Here's how the part is built. I have some questions about the finished solid (model axes, mm). Face numbers are marked on the shaded views. A direction names the side the tool comes from. Coordinates: 2 decimals unless noted, no trailing zeros.
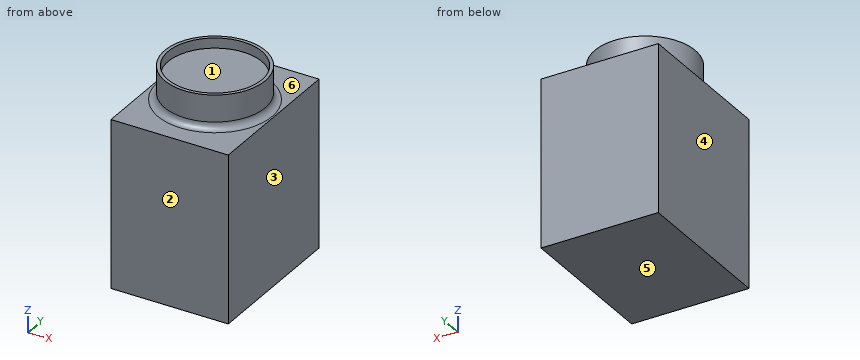
from build123d import *

# Parameters (mm, degrees)
SKETCH_W     = 35
SKETCH_H     = 45
PAD_DEPTH    = 50
SKETCH001_R  = 15
PAD001_DEPTH = 10
SKETCH002_R  = 14
POCKET_DEPTH = 3
FILLET_R     = 2


with BuildPart() as part:
    # Sketch → Pad (new body)
    with BuildSketch(Plane.XY):
        with Locations((2.787933, 6.169585)):
            Rectangle(SKETCH_W, SKETCH_H)
    extrude(amount=PAD_DEPTH)

    # Sketch001 (on Face6 of Pad) → Pad001 (join)
    with BuildSketch(Plane.XY.offset(50)):
        with Locations((2.787933, 6.169585)):
            Circle(SKETCH001_R)
    extrude(amount=PAD001_DEPTH)

    # Sketch002 (on Face8 of Pad001) → Pocket (cut)
    with BuildSketch(Plane.XY.offset(60)):
        with Locations((2.787933, 6.169585)):
            Circle(SKETCH002_R)
    extrude(amount=-POCKET_DEPTH, mode=Mode.SUBTRACT)

    # Fillet
    fillet_edges = [part.edges().sort_by_distance(p)[0] for p in [
        (-12.212067, 6.169585, 50),
    ]]
    fillet(fillet_edges, radius=FILLET_R)


solid = part.part
1. If I drill on line 1 (Z direction, x = 9, y = 1); line 2 (Z direction, x = 8, y = 26); line 3 (X direction, y = 5.5, z = 53.5), over which ranges is the centre line in solid material (lowest first)?
2. On a 3-axis mill with a long thin cutter (end or side, diameter ignored), from which of +Z, -Z, +X, -X, +Y, -Y can I reach the whole of each face in a straight line? I mean the marked faces 5 and 6. Say none if no direction works.
3. Thinking about a two-plate mould opening in X: for the marked faces 1, 2, 3 and 4, which applies, pulls with the +X half, pulls with the -X half, needs draft (parallel to the pull), parting line crosses it, or undercut?
4. For pin 1 Ø10.5 at (x, y) = (-3, 7.5) entering from +Z, with a flat end and sliding along its axis, tell me the tip position at first contact or that it passes through.
Response values:
1. line 1: z = 0 to 57
1. line 2: z = 0 to 50
1. line 3: x = -12.2 to 17.77
2. face 5: -Z, +X, -X, +Y, -Y
2. face 6: +Z
3. face 1: undercut
3. face 2: needs draft
3. face 3: pulls with the +X half
3. face 4: pulls with the -X half
4. pin 1: stops at z = 57
